from build123d import *

# Parameters (mm, degrees)
BOSS_EXTRU_1_DEPTH = 2


with BuildPart() as part:
    # Esquisse2 → Boss.-Extru.1 (new body)
    with BuildSketch(Plane.XY):
        Polygon((68.597300567, 260.777491871), (-336.373262181, 260.777491871), (-389.887980807, 207.262773245), (-389.887980807, 184.777491871), (-289.887980807, 184.777491871), (-289.887980807, 120.777491871), (-389.887980807, 120.777491871), (-389.887980807, -46.168159055), (-289.887980807, -46.168159055), (-289.887980807, -110.168159055), (-389.887980807, -110.168159055), (-389.887980807, -127.707789503), (-336.373262181, -181.222508129), (68.597300567, -181.222508129), (122.112019193, -127.707789503), (122.112019193, -46.168159055), (122.112019193, 120.777491871), (122.112019193, 207.262773245), align=None)
        Polygon((110.112019193, 120.777491871), (-27.887980807, 120.777491871), (-27.887980807, 188.777491871), (110.112019193, 188.547731592), align=None, mode=Mode.SUBTRACT)
        Polygon((-27.887980807, -114.168159055), (-27.887980807, -46.168159055), (110.112019193, -46.168159055), (110.112019193, -113.938398776), align=None, mode=Mode.SUBTRACT)
    extrude(amount=BOSS_EXTRU_1_DEPTH)


solid = part.part
Geometry: final body of the model. Coordinates: model frame, mm. Coordinates: 2 decimals unless noted, no trailing zeros. Order: outer loops, then holes, each group sorted by start corner. A loop starts at its lowest first (then second) coordinate and runs counter-clockwise, first axis right, second up.
1) Section A-A (y = 153). Return loops of the section in (x, z), then the cut area to 3 significant figures.
Result sheet:
outline: (-289.89, 0) - (-27.89, 0) - (-27.89, 2) - (-289.89, 2) - close; (110.11, 0) - (122.11, 0) - (122.11, 2) - (110.11, 2) - close
area: 548 mm2
2) Section D-D (y = -145). Return loops of the section in (x, z), then the cut area to 3 significant figures.
Result sheet:
outline: (-372.6, 0) - (104.82, 0) - (104.82, 2) - (-372.6, 2) - close
area: 955 mm2
3) Section B-B (z = 0.4). Return loops of the section in (x, y).
Result sheet:
outline: (-389.89, -127.71) - (-336.37, -181.22) - (68.6, -181.22) - (122.11, -127.71) - (122.11, 207.26) - (68.6, 260.78) - (-336.37, 260.78) - (-389.89, 207.26) - (-389.89, 184.78) - (-289.89, 184.78) - (-289.89, 120.78) - (-389.89, 120.78) - (-389.89, -46.17) - (-289.89, -46.17) - (-289.89, -110.17) - (-389.89, -110.17) - close; hole (-27.89, -114.17) - (110.11, -113.94) - (110.11, -46.17) - (-27.89, -46.17) - close; hole (-27.89, 120.78) - (110.11, 120.78) - (110.11, 188.55) - (-27.89, 188.78) - close
4) Draft query along Z for faces 1 (the flat face through (-362.76, 234.39, 0.99)), 2 (the flat face through (-137, 43, 2)), 3 (the flat face through (-137, 43, 0)). Return one class per face: released by +Z, released by -Z, zero draft, split by the parting line, or undercut.
Result sheet:
face 1: zero draft
face 2: released by +Z
face 3: released by -Z
5) Ray query, probe 1 along Y at (x, z) = (-2.5, 1.35); probe 2 along Y at (x, z) = (-291.5, 0.65); probe 3 along X at (y, z) = (-56.5, 1.45). Return the intervals inside material, ascending.
Result sheet:
probe 1: y = -181.22 to -114.13, -46.17 to 120.78, 188.74 to 260.78
probe 2: y = -181.22 to -110.17, -46.17 to 120.78, 184.78 to 260.78
probe 3: x = -289.89 to -27.89, 110.11 to 122.11
6) Section C-C (x = 26). Return loops of the section in (y, z), then the cut area to 3 significant figures.
Result sheet:
outline: (-181.22, 0) - (-114.08, 0) - (-114.08, 2) - (-181.22, 2) - close; (-46.17, 0) - (120.78, 0) - (120.78, 2) - (-46.17, 2) - close; (188.69, 0) - (260.78, 0) - (260.78, 2) - (188.69, 2) - close
area: 612 mm2
7) First-contact query: P1, Ø1, axis at x = -347, z = 1, coming from the -Y side; P2, Ø0.6, axis at x = -337.5, z = 1, coming from the -Y side; P3, Ø0.6, axis at y = -79, z = 1.5, coming from the -X side. Flat tips, straight axial feed; report the tip coordinate or a pass-through.
Result sheet:
P1: stops at y = -171.1
P2: stops at y = -180.4
P3: stops at x = -289.89
